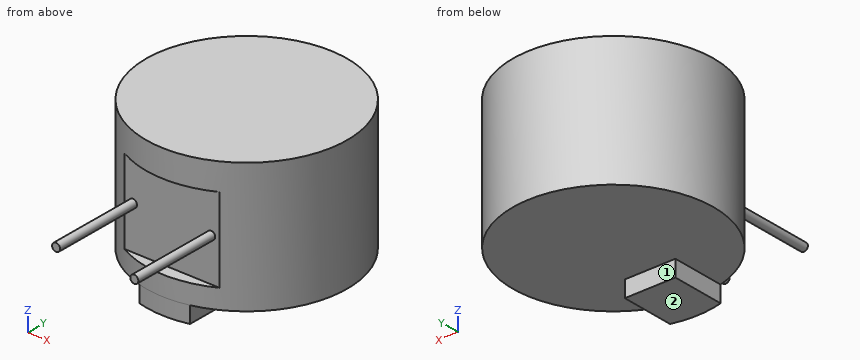
from build123d import *

# Parameters (mm, degrees)
SKETCH1_R           = 75
BOSS_EXTRUDE1_DEPTH = 97
CUT_EXTRUDE1_START  = -62.5
CUT_EXTRUDE1_DEPTH  = 62.5
SKETCH3_R           = 3
BOSS_EXTRUDE2_DEPTH = 68
BOSS_EXTRUDE3_START = 12.25
SKETCH4_W           = 37.85
SKETCH4_H           = 40
BOSS_EXTRUDE3_DEPTH = 12.25


with BuildPart() as part:
    # Sketch1 → Boss-Extrude1 (new body)
    with BuildSketch(Plane.XY):
        with Locations(Location((0, 0, 0), (0, 0, 180))):
            Circle(SKETCH1_R)
    extrude(amount=BOSS_EXTRUDE1_DEPTH)

    # Sketch2 → Cut-Extrude1 (cut)
    with BuildSketch(Plane(origin=(0, 0, 14.5), x_dir=(-1, 0, 0), z_dir=(0, 0, -1)).offset(CUT_EXTRUDE1_START)):
        Polygon((404.05546865, -66), (35.623026261, -66), (-35.623026261, -66), (-404.05546865, -66), (-404.05546865, -802.864884777), (404.05546865, -802.864884777), align=None)
    extrude(amount=CUT_EXTRUDE1_DEPTH, mode=Mode.SUBTRACT)

    # Sketch3 → Boss-Extrude2 (add)
    with BuildSketch(Plane.XZ.offset(66)):
        with Locations(Location((-29.25, 46.5, 0), (0, 0, 90))):
            Circle(SKETCH3_R)
        with Locations(Location((29.25, 46.5, 0), (0, 0, 90))):
            Circle(SKETCH3_R)
    extrude(amount=BOSS_EXTRUDE2_DEPTH)

    # Sketch4 → Boss-Extrude3 (add)
    with BuildSketch(Plane(origin=(0, 0, 0), x_dir=(-1, 0, 0), z_dir=(0, 0, -1)).offset(BOSS_EXTRUDE3_START)):
        with Locations((0, -52.573027875)):
            Rectangle(SKETCH4_W, SKETCH4_H)
        with BuildLine():
            Line((18.925, -72.573027875), (-18.925, -72.573027875))
            ThreePointArc((-18.925, -72.573027875), (0, -75), (18.925, -72.573027875))
        make_face()
    extrude(amount=-BOSS_EXTRUDE3_DEPTH)


solid = part.part
Build history of the part. All positions in model axes, mm. Face numbers are marked on the shaded views. A direction names the side the tool comes from. Round coordinates to 2 decimals unless told otherwise and drop trailing zeros. Write each loop counter-clockwise with the first axis right and the second up, starting at its lowest first coordinate (ties: lowest second). Pieces come first, ordered by that corner, then holes. Notation, with made-up numbers: M 27.5,-22.5 L 69.5,-22.5 A13 cw 69.5,-4.5 Z; hole C 13.5,5.25 d10. An arc over 180 degrees is marked long. Use CSV: the item, a comma, the result in double quotes.
1. Saw through at A-A (x = 0). Give the cut face in (y, z), plus the area to 3 significant figures.
Reply:
outline,"M -75,-12.25 L -32.57,-12.25 L -32.57,0 L 75,0 L 75,97 L -75,97 L -75,77 L -66,77 L -66,14.5 L -75,14.5 Z"
area,"14,500 mm²"
2. Saw through at B-B (z = 46.5). Give the cut face in (x, y), plus the area to 3 significant figures.
Reply:
outline,"M -35.62,-66 L -32.25,-66 L -32.25,-134 L -26.25,-134 L -26.25,-66 L 26.25,-66 L 26.25,-134 L 32.25,-134 L 32.25,-66 L 35.62,-66 A75 ccw long Z"
area,"18,100 mm²"
3. Tool access for the marked faces 1 and 2: list every direction of +Z, -Z, +X, -X, +Y, -Y with a clear straight run to the whole face (end or side of a thin tool).
Reply:
face 1,"-Z, +X, -X, +Y"
face 2,"-Z, +X, -X, +Y, -Y"
4. Saw through at C-C (y = 0). Give the cut face in (x, z), plus the area to 4 significant figures.
Reply:
outline,"M -75,0 L 75,0 L 75,97 L -75,97 Z"
area,"14,550 mm²"
5. Wall check: probe 1 along Y at (x, z) = (2, -4.5); probe 2 along Z at (x, y) = (32, -17); probe 3 along X at (y, z) = (1, 56). Give the ranges that are in metal, low to high. Write a range as from..to.
Reply:
probe 1,"y = -74.97..-32.57"
probe 2,"z = 0..97"
probe 3,"x = -74.99..74.99"
6. Flat gauge pins, fed straight in: pin 1 (10 mm diameter, centred on y = -49.5, z = -7.5, fed in from +X) (3 decimals); pin 2 (2 mm diameter, centred on x = 26, y = -103, fed in from +Z); pin 3 (6 mm diameter, centred on x = 47, z = 70, fed in from -Y); pin 4 (4 mm diameter, centred on y = -88, z = 40.5, fed in from +X). Where does each tip first touch, or does it go through?
Reply:
pin 1,"stops at x = 18.925"
pin 2,"stops at z = 48.48"
pin 3,"stops at y = -60.74"
pin 4,"passes through"
7. Saw through at D-D (x = 29.25). Give the cut face in (y, z), plus the area to 3 significant figures.
Reply:
outline,"M -134,43.5 L -66,43.5 L -66,14.5 L -69.06,14.5 L -69.06,0 L 69.06,0 L 69.06,97 L -69.06,97 L -69.06,77 L -66,77 L -66,49.5 L -134,49.5 Z"
area,"13,600 mm²"
